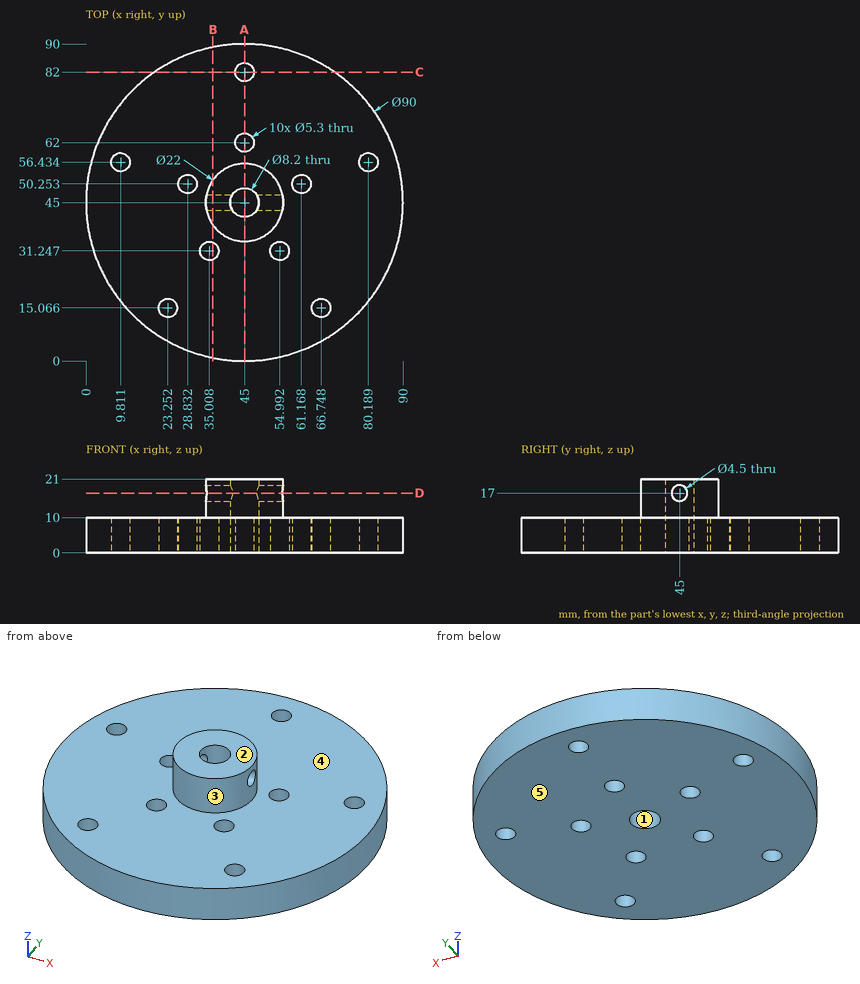
Could you check a few things on this drawing? It's one solid part, dimensions in mm from its lowest x, y, z. A direction names the side the tool comes from. Give positions to 0.01 mm unless a question says otherwise; leave off trailing zeros. Loops run counter-clockwise (first coordinate to the right, second up) from the corner with the lowest first, then second, coordinate; pieces in that order, holes last. Notation, with made-up numbers: M 78.5,0.25 L 136.5,0.25 A15 ccw 136.5,14.25 Z; hole C -32,85 d4. An arc over 180 degrees is marked long. One line per question, with ' | ' between items. Start each with the question number.
Q1. If we section it at C-C (y = 82): Please give me the cut outline in (x, z).
Q2. If we section it at B-B (x = 36): State how many separate pieces and enclosed holes the cut face has, plus the area to 3 significant figures.
Q3. For pin 1 Ø7 at (x, y) = (45, 62) entering from +Z; pin 2 Ø10 at (y, z) = (43, 18.5) entering from -X; pin 3 Ø12 at (x, z) = (40, 10) entering from +Y, each with a flat end and sliding along its axis, tell me the tip position at first contact or that it passes through.
Q4. If we mould it in two halves opening along X, with no side actions, what happens to the marked faces 1, 2 and 3? For each: +X half, -X half, draft (parallel to the pull), parting line (faces both ways), or undercut.
Q5. If we section it at A-A (x = 45): Please give me the cut outline in (y, z), plus the area to 3 significant figures.
Q6. If we section it at D-D (z = 17): Please give me the cut outline in (x, y), plus the area to 3 significant figures.
Q7. For the marked faces 4 and 5, which set-ups out of +Z, -Z, +X, -X, +Y, -Y let a thin tool reach every point of the face, with its end or its side?
Q8. If I drill on line 1 (Y direction, x = 45, z = 5); line 2 (Z direction, x = 83, y = 22.5); line 3 (X direction, y = 52, z = 4.25) (1 decimal), over which ranges is the centre line in solid material (lowest first)? Write a range as from..to.
Computed:
1) outline: M 19.39,0 L 42.35,0 L 42.35,10 L 19.39,10 Z; M 47.65,0 L 70.61,0 L 70.61,10 L 47.65,10 Z
2) separate pieces: 2 | enclosed holes: 1 | area: 956 mm²
3) pin 1: stops at z = 10 | pin 2: stops at x = 34 | pin 3: stops at y = 90
4) face 1: undercut | face 2: draft | face 3: parting line
5) outline: M 0,0 L 40.9,0 L 40.9,21 L 34,21 L 34,10 L 0,10 Z; M 49.1,0 L 59.35,0 L 59.35,10 L 56,10 L 56,21 L 49.1,21 Z; M 64.65,0 L 79.35,0 L 79.35,10 L 64.65,10 Z; M 84.65,0 L 90,0 L 90,10 L 84.65,10 Z | area: 864 mm²
6) outline: M 34.23,42.75 A11 ccw 55.77,42.75 L 48.43,42.75 A4.1 cw 41.57,42.75 Z; M 34.23,47.25 L 41.57,47.25 A4.1 cw 48.43,47.25 L 55.77,47.25 A11 ccw Z | area: 264 mm²
7) face 4: +Z | face 5: -Z, +X, -X, +Y, -Y
8) line 1: y = 0..40.9, 49.1..59.35, 64.65..79.35, 84.65..90 | line 2: z = 0..10 | line 3: x = 0.5..26.8, 30.8..59.2, 63.2..89.5
